Solid Edge part; units mm, degrees
sketch "Sketch1" plane through (0, 0, 0) normal (0, 0, 1) x (1, 0, 0)
  circle A0 centre (0, 0) radius 18.5
extrude "Protrusion1" add sketch "Sketch1" against normal blind 4
sketch "Sketch2" plane through (0, 0, -4) normal (0, 0, -1) x (0, 1, 0)
  circle A0 centre (0, 0) radius 23.5
extrude "Extrusionsausprägung_3" add sketch "Sketch2" along normal blind 3
hole "Bohrung_1" at (0, -8.376, 0) direction (0, 0, -1) diameter 6 end up to next
hole "Hole1" at (0, 8.376, 0) direction (0, 0, -1) diameter 6 end up to next
sketch "Sketch3" plane through (0, 0, -7) normal (0, 0, -1) x (0, -1, 0)
  line L0 (-11.376, 9.25) -> (-11.376, -9.25)
  line L1 (-11.376, -9.25) -> (-5.376, -9.25)
  line L2 (-5.376, -9.25) -> (-5.376, 9.25)
  line L3 (-5.376, 9.25) -> (-11.376, 9.25)
  line L4 (5.376, -9.25) -> (5.376, 9.25)
  line L5 (5.376, 9.25) -> (11.376, 9.25)
  line L6 (11.376, 9.25) -> (11.376, -9.25)
  line L7 (11.376, -9.25) -> (5.376, -9.25)
extrude "Extrusionsausschnitt_2" cut sketch "Sketch3" against normal blind 4
sketch "Sketch4" plane through (0.0615, 0.1775, 0) normal (0, 0, 1) x (0, 1, 0)
  arc A0 (4.0837, 23.8834) -> (10.2705, 21.8899) centre (-0.1775, 0.0615) cw
  line L0 (8.5013, 16.3994) -> (10.2705, 21.8899)
  arc A1 (2.3146, 18.3929) -> (8.5013, 16.3994) centre (-0.1775, 0.0615) cw
  line L1 (4.0837, 23.8834) -> (2.3146, 18.3929)
  arc A2 (-24.0388, 4.0967) -> (-22.104, 10.3021) centre (-0.1775, 0.0615) cw
  line L2 (-16.597, 8.5851) -> (-22.104, 10.3021)
  arc A3 (-18.5317, 2.3797) -> (-16.597, 8.5851) centre (-0.1775, 0.0615) cw
  line L3 (-24.0388, 4.0967) -> (-18.5317, 2.3797)
  arc A4 (-4.1106, -23.8167) -> (-10.3242, -21.9086) centre (-0.1775, 0.0615) cw
  line L4 (-8.6308, -16.3942) -> (-10.3242, -21.9086)
  arc A5 (-2.4172, -18.3024) -> (-8.6308, -16.3942) centre (-0.1775, 0.0615) cw
  line L5 (-4.1106, -23.8167) -> (-2.4172, -18.3024)
  arc A6 (24.0225, 0.0615) -> (23.1495, -6.3796) centre (-0.1775, 0.0615) cw
  line L6 (17.4333, -5.6049) -> (23.1495, -6.3796)
  arc A7 (18.3062, 0.8362) -> (17.4333, -5.6049) centre (-0.1775, 0.0615) cw
  line L7 (24.0225, 0.0615) -> (18.3062, 0.8362)
extrude "Protrusion2" add sketch "Sketch4" against normal blind 9
sketch "Sketch5" plane through (0.0282, 0.1694, 0) normal (0, 0, 1) x (-0.9518, 0.3067, 0)
  circle A0 centre (-0.0251, 0.1699) radius 30
  circle A1 centre (-0.0251, 0.1699) radius 23.5
extrude "Cutout1" cut sketch "Sketch5" against normal through all
Part model, mm, in its own coordinate system. A direction names the side the tool comes from. Round coordinates to 2 decimals unless told otherwise and drop trailing zeros. Order: outer loops, then holes, each group sorted by start corner. A loop starts at its lowest first (then second) coordinate and runs counter-clockwise, first axis right, second up. Notation, with made-up numbers: M 6,-38.5 L 55,-38.5 A13 cw 55,-30.5 Z; hole C 42,-5 d8. An arc over 180 degrees is marked long. Answer in a Markdown table with one row per item. Add a question column.
Q1. Cut at D-D on x = -4.5. Give the cut face in (y, z), and give its area (3 significant figures).
Q2. Cut at C-C on x = -13.5. Give the cut face in (y, z), and give its area (3 significant figures).
Q3. 3-axis set-ups, long thin cutter, end or side, ignore diameter. For faces 1 (the face through (-18.713, 9.444, -3.437)), 2 (the face through (-16.495, -8.376, -1.972)), 3 (the face through (-6, 8, -3)), 4 (the face through (-0.43, 21.03, -1.97)): which of +Z, -Z, +X, -X, +Y, -Y reach the whole face in a straight line?
Q4. Cut at B-B on y = 8. Give the cut face in (x, z).
Q5. Mould opens along Y. For faces 5 (the face through (6, 20.08, -1.97)), 6 (the face through (-11, 17, -4)), 7 (the face through (-6, -8, -3)), 8 (the face through (-0.43, 21.03, -7.99)) say: +Y half, -Y half, draft (parallel to the pull), parting line (faces both ways), or undercut.
Q6. Wall check: L1, parallel to Y at x = 0, z = -1.8; L2, parallel to Y at x = -4.5, z = -4.75; L3, parallel to X at y = 9, z = -6.5. Give the ranges that are in metal, low to high. Write a range as from..to.
Q7. Cut at A-A on z = -1.25. Give the cut face in (x, y), and give its area (3 significant figures).
Q8. Pin check, flat tips, straight feed: pin 1 (1.8 mm diameter, centred on x = -2.5, y = 7.5, fed in from -Z); pin 2 (4.5 mm diameter, centred on y = 8.5, z = -4, fed in from -X); pin 3 (1.5 mm diameter, centred on y = 13.5, z = -2, fed in from +X). Stop position of each tip, or through.
Established:
| question | item | result |
|---|---|---|
| 1 | outline | M -23.07,-9 L -17.94,-9 L -17.94,-7 L -11.38,-7 L -11.38,-3 L -5.38,-3 L -5.38,-7 L 5.38,-7 L 5.38,-3 L 11.38,-3 L 11.38,-7 L 23.07,-7 L 23.07,-4 L 17.94,-4 L 17.94,0 L -23.07,0 Z |
| 1 | area | 265 mm2 |
| 2 | outline | M -19.24,-7 L 19.24,-7 L 19.24,-4 L 12.65,-4 L 12.65,0 L -12.65,0 L -12.65,-4 L -19.24,-4 Z |
| 2 | area | 217 mm2 |
| 3 | face 1 | +Z, +Y |
| 3 | face 2 | +Z, -X |
| 3 | face 3 | -Z |
| 3 | face 4 | +Z, -X, +Y |
| 4 | outline | M -22.1,-9 L -16.68,-9 L -16.68,-7 L -9.25,-7 L -9.25,-3 L -2.98,-3 L -2.98,0 L -22.1,0 Z; M 2.98,-3 L 9.25,-3 L 9.25,-7 L 22.1,-7 L 22.1,-4 L 16.68,-4 L 16.68,0 L 2.98,0 Z |
| 5 | face 5 | undercut |
| 5 | face 6 | draft |
| 5 | face 7 | undercut |
| 5 | face 8 | +Y half |
| 6 | L1 | y = -18.5..-11.38, -5.38..5.38, 11.38..23.5 |
| 6 | L2 | y = -23.07..-11.38, -5.38..5.38, 11.38..23.07 |
| 6 | L3 | x = -21.71..-9.25, 9.25..21.71 |
| 7 | outline | M -23.15,4.04 L -18.33,2.49 A18.5 ccw -8.52,-16.42 L -10.03,-21.25 A23.5 ccw -3.82,-23.19 L -2.32,-18.35 A18.5 ccw 16.46,-8.45 L 21.29,-9.94 A23.5 ccw 23.2,-3.73 L 18.36,-2.24 A18.5 ccw 5.67,17.61 L 6.35,22.63 A23.5 ccw -0.09,23.5 L -0.77,18.48 A18.5 ccw -16.34,8.68 L -21.16,10.23 A23.5 ccw Z; hole C 0,-8.38 d6; hole C 0,8.38 d6 |
| 7 | area | 1,150 mm2 |
| 8 | pin 1 | stops at z = -3 |
| 8 | pin 2 | stops at x = -22.65 |
| 8 | pin 3 | stops at x = 13.4 |
